Part print with two shaded views. Sizes in mm from the minimum x, y, z corner. A direction names the side the tool comes from. Round coordinates to 2 decimals unless told otherwise and drop trailing zeros. Order: outer loops, then holes, each group sorted by start corner. A loop starts at its lowest first (then second) coordinate and runs counter-clockwise, first axis right, second up. Notation, with made-up numbers: (71.5, 31.5) -> (85.5, 31.5) arc R29 cw to (85.5, 57.5) -> close; hole circle Ø6 at (-39.5, 73). An arc over 180 degrees is marked (long way). Use a Markdown table: item, result. Add a question column.
Item 1: Slice it at D-D, the plane z = 15.5. Give the cut face in (x, y), plus the area to 3 significant figures.
Item 2: Slice it at A-A, the plane y = 10. Give the cut face in (x, z) (1 decimal).
Item 3: Slice it at C-C, the plane y = 14.5. Give the cut face in (x, z) (1 decimal).
Item 4: Probe L1, parallel to Z at x = 14.5, y = 19; L2, parallel to Z at x = 40, y = 14.5; L3, parallel to Y at x = 18, z = 31 (1 decimal). List the from-to ranges inside material, lowest first.
Item 5: Pin check, flat tips, straight feed: pin 1 (1.5 mm diameter, centred on x = 49, z = 28, fed in from -Y); pin 2 (5 mm diameter, centred on y = 22, z = 21, fed in from +X) (1 decimal); pin 3 (1.5 mm diameter, centred on x = 13.5, z = 39.5, fed in from -Y). Stop position of each tip, or through.
Item 6: Slice it at B-B, the plane x = 37. Give the cut face in (y, z) (1 decimal).
Item 7: 3-axis set-ups, long thin cutter, end or side, ignore diameter. For the marked faces 1 and 2: which of +Z, -Z, +X, -X, +Y, -Y reach the whole face in a straight line?
Item 8: Two-plate mould, pull along Z, no slides. Class the marked faces 3, 4 and 5: released by +Z, released by -Z, zero draft, split by the parting line, or undercut.
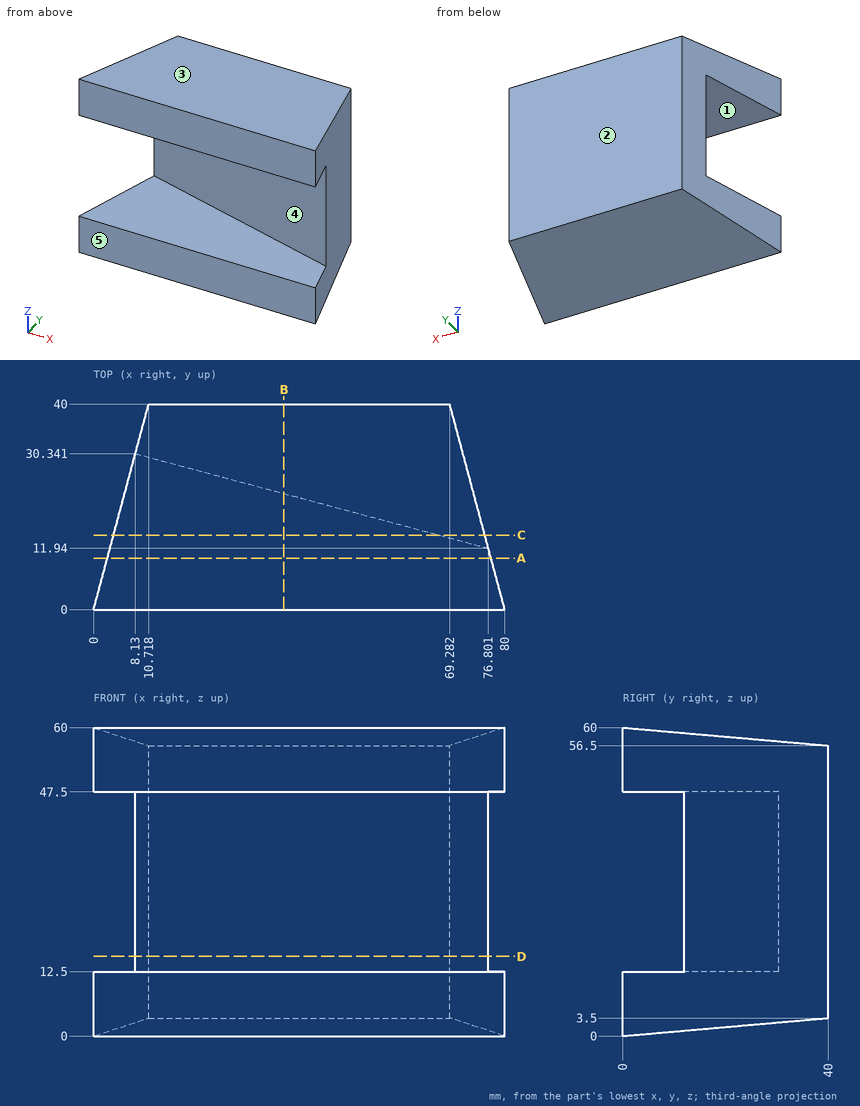
Check sheet entries:
| question | item | result |
|---|---|---|
| 1 | outline | (8.13, 30.34) -> (76.8, 11.94) -> (69.28, 40) -> (10.72, 40) -> close |
| 1 | area | 1,180 mm2 |
| 2 | outline | (2.7, 0.9) -> (77.3, 0.9) -> (77.3, 12.5) -> (2.7, 12.5) -> close; (2.7, 47.5) -> (77.3, 47.5) -> (77.3, 59.1) -> (2.7, 59.1) -> close |
| 3 | outline | (3.9, 1.3) -> (76.1, 1.3) -> (76.1, 58.7) -> (3.9, 58.7) -> (3.9, 47.5) -> (67.2, 47.5) -> (67.2, 12.5) -> (3.9, 12.5) -> close |
| 4 | L1 | 1.66 to 12.5, 47.5 to 58.34 |
| 4 | L2 | 1.27 to 12.5, 47.5 to 58.73 |
| 4 | L3 | 27.7 to 40 |
| 5 | pin 1 | y = 19.19 |
| 5 | pin 2 | x = 74.8 |
| 5 | pin 3 | y = 28.7 |
| 6 | outline | (0, 0) -> (40, 3.5) -> (40, 56.5) -> (0, 60) -> (0, 47.5) -> (22.6, 47.5) -> (22.6, 12.5) -> (0, 12.5) -> close |
| 7 | face 1 | -X, -Y |
| 7 | face 2 | +Z, -Z, +X, -X, +Y |
| 8 | face 3 | released by +Z |
| 8 | face 4 | undercut |
| 8 | face 5 | zero draft |
